Source: CAD feature listing. Evaluate the final solid. Frame: model axes, mm. Face numbers are marked on the shaded views. Give positions to 0.01 mm unless a question says otherwise; leave off trailing zeros. Loops run counter-clockwise (first coordinate to the right, second up) from the corner with the lowest first, then second, coordinate; pieces in that order, holes last.
from build123d import *

# Parameters (mm, degrees)
SKETCH3_R           = 21
BOSS_EXTRUDE2_DEPTH = 2
SKETCH4_R           = 10.05
CUT_EXTRUDE2_DEPTH  = 12.5
SKETCH5_R           = 21
BOSS_EXTRUDE3_DEPTH = 24
SKETCH6_R           = 20
CUT_EXTRUDE3_DEPTH  = 24
SKETCH7_R           = 21
BOSS_EXTRUDE4_DEPTH = 12.5
SKETCH8_R           = 10.05
CUT_EXTRUDE4_DEPTH  = 12.5
SKETCH9_R           = 21
BOSS_EXTRUDE5_DEPTH = 19
SKETCH10_R          = 20
CUT_EXTRUDE5_DEPTH  = 19
SKETCH11_R          = 21
BOSS_EXTRUDE6_DEPTH = 14.5
SKETCH12_R          = 7.5
CUT_EXTRUDE6_DEPTH  = 14.5
SKETCH13_R          = 21
BOSS_EXTRUDE7_DEPTH = 75
SKETCH14_R          = 20
CUT_EXTRUDE7_DEPTH  = 75
CHAMFER7_SIZE       = 11
CHAMFER8_SIZE       = 12.5


# Some blends are built 0.0001 mm under size
with BuildPart() as part:
    # Sketch3 → Boss-Extrude2 (new body)
    with BuildSketch(Plane(origin=(0, 0, 0), x_dir=(1, 0, 0), z_dir=(0, 1, 0))):
        with Locations(Location((0, 0, 0), (0, 0, 270))):
            Circle(SKETCH3_R)
    extrude(amount=BOSS_EXTRUDE2_DEPTH)

    # Sketch4 → Cut-Extrude2 (cut)
    with BuildSketch(Plane(origin=(0, 2, 0), x_dir=(1, 0, 0), z_dir=(0, 1, 0))):
        with Locations(Location((0, 0, 0), (0, 0, 270))):
            Circle(SKETCH4_R)
    extrude(amount=-CUT_EXTRUDE2_DEPTH, mode=Mode.SUBTRACT)

    # Sketch5 → Boss-Extrude3 (add)
    with BuildSketch(Plane(origin=(0, 2, 0), x_dir=(1, 0, 0), z_dir=(0, 1, 0))):
        with Locations(Location((0, 0, 0), (0, 0, 270))):
            Circle(SKETCH5_R)
    extrude(amount=BOSS_EXTRUDE3_DEPTH)

    # Sketch6 → Cut-Extrude3 (cut)
    with BuildSketch(Plane(origin=(0, 26, 0), x_dir=(1, 0, 0), z_dir=(0, 1, 0))):
        with Locations(Location((0, 0, 0), (0, 0, 270))):
            Circle(SKETCH6_R)
    extrude(amount=-CUT_EXTRUDE3_DEPTH, mode=Mode.SUBTRACT)

    # Sketch7 → Boss-Extrude4 (add)
    with BuildSketch(Plane(origin=(0, 26, 0), x_dir=(1, 0, 0), z_dir=(0, 1, 0))):
        with Locations(Location((0, 0, 0), (0, 0, 270))):
            Circle(SKETCH7_R)
    extrude(amount=BOSS_EXTRUDE4_DEPTH)

    # Sketch8 → Cut-Extrude4 (cut)
    with BuildSketch(Plane(origin=(0, 38.5, 0), x_dir=(1, 0, 0), z_dir=(0, 1, 0))):
        with Locations(Location((0, 0, 0), (0, 0, 270))):
            Circle(SKETCH8_R)
    extrude(amount=-CUT_EXTRUDE4_DEPTH, mode=Mode.SUBTRACT)

    # Sketch9 → Boss-Extrude5 (add)
    with BuildSketch(Plane(origin=(0, 38.5, 0), x_dir=(1, 0, 0), z_dir=(0, 1, 0))):
        with Locations(Location((0, 0, 0), (0, 0, 270))):
            Circle(SKETCH9_R)
    extrude(amount=BOSS_EXTRUDE5_DEPTH)

    # Sketch10 → Cut-Extrude5 (cut)
    with BuildSketch(Plane(origin=(0, 57.5, 0), x_dir=(1, 0, 0), z_dir=(0, 1, 0))):
        with Locations(Location((0, 0, 0), (0, 0, 270))):
            Circle(SKETCH10_R)
    extrude(amount=-CUT_EXTRUDE5_DEPTH, mode=Mode.SUBTRACT)

    # Sketch11 → Boss-Extrude6 (add)
    with BuildSketch(Plane(origin=(0, 57.5, 0), x_dir=(1, 0, 0), z_dir=(0, 1, 0))):
        with Locations(Location((0, 0, 0), (0, 0, 270))):
            Circle(SKETCH11_R)
    extrude(amount=BOSS_EXTRUDE6_DEPTH)

    # Sketch12 → Cut-Extrude6 (cut)
    with BuildSketch(Plane(origin=(0, 72, 0), x_dir=(1, 0, 0), z_dir=(0, 1, 0))):
        with Locations(Location((0, 0, 0), (0, 0, 270))):
            Circle(SKETCH12_R)
    extrude(amount=-CUT_EXTRUDE6_DEPTH, mode=Mode.SUBTRACT)

    # Sketch13 → Boss-Extrude7 (add)
    with BuildSketch(Plane(origin=(0, 72, 0), x_dir=(1, 0, 0), z_dir=(0, 1, 0))):
        with Locations(Location((0, 0, 0), (0, 0, 270))):
            Circle(SKETCH13_R)
    extrude(amount=BOSS_EXTRUDE7_DEPTH)

    # Sketch14 → Cut-Extrude7 (cut)
    with BuildSketch(Plane(origin=(0, 147, 0), x_dir=(1, 0, 0), z_dir=(0, 1, 0))):
        with Locations(Location((0, 0, 0), (0, 0, 270))):
            Circle(SKETCH14_R)
    extrude(amount=-CUT_EXTRUDE7_DEPTH, mode=Mode.SUBTRACT)

    # Chamfer7
    # the kernel refuses this chamfer: 11 mm, written as the material it takes off along each edge
    with BuildSketch(Plane(origin=(0, 26, 0), x_dir=(0, 0, 1), z_dir=(-1, 0, 0))) as chamfer7_piece_1_section:
        Polygon((10.05 + CHAMFER7_SIZE, 0), (10.05, CHAMFER7_SIZE), (10.05, 0), align=None)
    chamfer7_piece_1 = revolve(axis=Axis((0, 26, 0), (0, 1, 0)), mode=Mode.PRIVATE)
    chamfer7_piece_1 = chamfer7_piece_1 & Plane(origin=(0, 32.05519731, 0), x_dir=(0, 0, 1), z_dir=(0, 1, 0)) * Cylinder(20, 85, mode=Mode.PRIVATE)
    add(chamfer7_piece_1, mode=Mode.SUBTRACT)

    # Chamfer8
    chamfer8_edges = [part.edges().sort_by_distance(p)[0] for p in [
        (0, 57.5, -7.5),
    ]]
    chamfer(chamfer8_edges, length=CHAMFER8_SIZE - 0.0001)  # a hair under: the kernel refuses the full size


solid = part.part
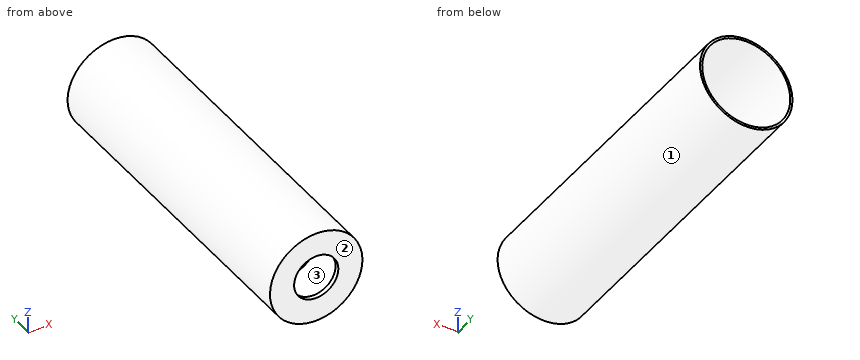
1) Cut plane D-D (x = -13.5). State how many separate pieces and enclosed holes the cut face has, and give its area (3 significant figures).
Checks:
separate pieces: 1
enclosed holes: 2
area: 970 mm2
2) Contact query for flat-ended pins moving along their axis: P1, Ø4, axis at x = 4.5, y = 119.5, coming from the -Z side; P2, Ø12, axis at x = 3, z = -4, coming from the +Y side; P3, Ø2, axis at x = -16.5, y = 29.5, coming from the +Z side; P4, Ø10, axis at x = -14, z = 8.5, coming from the -Y side. Output: stop coordinate, or through.
Checks:
P1: stops at z = -20.85
P2: stops at y = 72
P3: stops at z = 14.17
P4: stops at y = 0
3) Cut plane C-C (y = 34). Return loops of the section in (x, z).
Checks:
outline: circle Ø42 at (0, 0); hole circle Ø26.1 at (0, 0)
4) Pull-direction query (X, two-part tool) for the marked faces 1, 2 and 3; classes: released by +X, released by -X, zero draft, split by the parting line, or undercut.
Checks:
face 1: split by the parting line
face 2: zero draft
face 3: undercut
5) Ray query, probe 1 along Y at (x, z) = (-12, -15); probe 2 along X at (y, z) = (93, 0); probe 3 along Y at (x, z) = (-12.5, -15). Return the intervals inside material, ascending.
Checks:
probe 1: y = 0 to 2, 27.84 to 38.5, 58.29 to 72
probe 2: x = -21 to -20, 20 to 21
probe 3: y = 0 to 2, 27.52 to 38.5, 57.97 to 72
